Here's how the part is built. I have some questions about the finished solid (model axes, mm). Round coordinates to 2 decimals unless told otherwise and drop trailing zeros. Write item = value, one per line. Start each with the question number.
(1) Will these pins go through, and if not, where does the flat tip stop? pin 1 Ø0.7 at (y, z) = (-0.5, 132.5) entering from -X; pin 2 Ø0.6 at (y, z) = (9, 109) entering from -X; pin 3 Ø1.1 at (y, z) = (0, 100.5) entering from +X.
(2) If we mould it in two halves opening along Y, with no side actions, what happens to faces 1 (the flat face through (-0.1, 2.4, 256.86)), 2 (the cylindrical face through (-1.706, -1.308, 126.632)), 3 (the flat face through (-6, -10, 127))? For each: released by +Y, released by -Y, zero draft, split by the parting line, or undercut.
(3) I need wall thicknesses on line 1 along Y through (x, z) = (3.5, 14.5); line 2 along X through (y, z) = (-4.75, 106); line 3 along X through (y, z) = (2.75, 139.5). Which ranges of each line are inside material? Lowest first, please.
```python
from build123d import *

# Parameters (mm, degrees)
BOSS_EXTRU_1_DEPTH = 256.86


with BuildPart() as part:
    # Esquisse1 → Boss.-Extru.1 (new body)
    with BuildSketch(Plane.XY):
        with BuildLine():
            Line((-3.255887446, 4.528679645), (-5.506192286, 6.778984485))
            ThreePointArc((-5.506192286, 6.778984485), (-5.686636441, 7.686138511), (-4.917588391, 8.199999989))
            Line((-4.917588391, 8.199999989), (-2.799999991, 8.199999989))
            ThreePointArc((-2.799999991, 8.199999989), (-2.587867957, 8.287867955), (-2.499999991, 8.499999989))
            Line((-2.499999991, 8.499999989), (-2.499999991, 9.199999989))
            ThreePointArc((-2.499999991, 9.199999989), (-2.734314566, 9.765685414), (-3.299999991, 9.999999989))
            Line((-3.299999991, 9.999999989), (-7.999999991, 9.999999989))
            ThreePointArc((-7.999999991, 9.999999989), (-9.414213554, 9.414213552), (-9.999999991, 7.999999989))
            Line((-9.999999991, 7.999999989), (-9.999999991, 3.299999989))
            ThreePointArc((-9.999999991, 3.299999989), (-9.765685416, 2.734314564), (-9.199999991, 2.499999989))
            Line((-9.199999991, 2.499999989), (-8.499999991, 2.499999989))
            ThreePointArc((-8.499999991, 2.499999989), (-8.287867957, 2.587867955), (-8.199999991, 2.799999989))
            Line((-8.199999991, 2.799999989), (-8.199999991, 4.917588389))
            ThreePointArc((-8.199999991, 4.917588389), (-7.686138517, 5.686636433), (-6.778984497, 5.506192279))
            Line((-6.778984497, 5.506192279), (-4.528679657, 3.255887439))
            ThreePointArc((-4.528679657, 3.255887439), (-3.878361403, 2.282617393), (-3.650000001, 1.134567096))
            Line((-3.650000001, 1.134567096), (-3.650000001, -1.134567114))
            ThreePointArc((-3.650000001, -1.134567114), (-3.878361403, -2.282617409), (-4.528679656, -3.255887454))
            Line((-4.528679656, -3.255887454), (-6.778984496, -5.506192294))
            ThreePointArc((-6.778984496, -5.506192294), (-7.686138522, -5.686636449), (-8.2, -4.9175884))
            Line((-8.2, -4.9175884), (-8.2, -2.8))
            ThreePointArc((-8.2, -2.8), (-8.287867966, -2.587867966), (-8.5, -2.5))
            Line((-8.5, -2.5), (-9.2, -2.5))
            ThreePointArc((-9.2, -2.5), (-9.765685425, -2.734314575), (-10, -3.3))
            Line((-10, -3.3), (-10, -8))
            ThreePointArc((-10, -8), (-9.414213562, -9.414213562), (-8, -10))
            Line((-8, -10), (-3.3, -10))
            ThreePointArc((-3.3, -10), (-2.734314575, -9.765685425), (-2.5, -9.2))
            Line((-2.5, -9.2), (-2.5, -8.5))
            ThreePointArc((-2.5, -8.5), (-2.587867966, -8.287867966), (-2.8, -8.2))
            Line((-2.8, -8.2), (-4.9175884, -8.2))
            ThreePointArc((-4.9175884, -8.2), (-5.686636444, -7.686138526), (-5.50619229, -6.778984506))
            Line((-5.50619229, -6.778984506), (-3.25588745, -4.528679666))
            ThreePointArc((-3.25588745, -4.528679666), (-2.282617404, -3.878361412), (-1.134567106, -3.650000009))
            Line((-1.134567106, -3.650000009), (1.134567104, -3.650000009))
            ThreePointArc((1.134567104, -3.650000009), (2.282617399, -3.878361412), (3.255887444, -4.528679664))
            Line((3.255887444, -4.528679664), (5.506192284, -6.778984504))
            ThreePointArc((5.506192284, -6.778984504), (5.686636439, -7.686138531), (4.917588389, -8.200000009))
            Line((4.917588389, -8.200000009), (2.799999989, -8.200000009))
            ThreePointArc((2.799999989, -8.200000009), (2.587867955, -8.287867974), (2.499999989, -8.500000009))
            Line((2.499999989, -8.500000009), (2.499999989, -9.200000009))
            ThreePointArc((2.499999989, -9.200000009), (2.734314564, -9.765685434), (3.299999989, -10.000000009))
            Line((3.299999989, -10.000000009), (7.999999989, -10.000000009))
            ThreePointArc((7.999999989, -10.000000009), (9.414213552, -9.414213571), (9.999999989, -8.000000009))
            Line((9.999999989, -8.000000009), (9.999999989, -3.300000009))
            ThreePointArc((9.999999989, -3.300000009), (9.765685414, -2.734314584), (9.199999989, -2.500000009))
            Line((9.199999989, -2.500000009), (8.499999989, -2.500000009))
            ThreePointArc((8.499999989, -2.500000009), (8.287867955, -2.587867974), (8.199999989, -2.800000009))
            Line((8.199999989, -2.800000009), (8.199999989, -4.917588409))
            ThreePointArc((8.199999989, -4.917588409), (7.686138515, -5.686636452), (6.778984495, -5.506192299))
            Line((6.778984495, -5.506192299), (4.528679655, -3.255887459))
            ThreePointArc((4.528679655, -3.255887459), (3.878361401, -2.282617412), (3.649999999, -1.134567115))
            Line((3.649999999, -1.134567115), (3.649999999, 1.134567095))
            ThreePointArc((3.649999999, 1.134567095), (3.878361401, 2.28261739), (4.528679654, 3.255887435))
            Line((4.528679654, 3.255887435), (6.778984494, 5.506192275))
            ThreePointArc((6.778984494, 5.506192275), (7.68613852, 5.68663643), (8.199999998, 4.917588381))
            Line((8.199999998, 4.917588381), (8.199999998, 2.799999981))
            ThreePointArc((8.199999998, 2.799999981), (8.287867964, 2.587867946), (8.499999998, 2.499999981))
            Line((8.499999998, 2.499999981), (9.199999998, 2.499999981))
            ThreePointArc((9.199999998, 2.499999981), (9.765685423, 2.734314556), (9.999999998, 3.299999981))
            Line((9.999999998, 3.299999981), (9.999999998, 7.999999981))
            ThreePointArc((9.999999998, 7.999999981), (9.41421356, 9.414213543), (7.999999998, 9.999999981))
            Line((7.999999998, 9.999999981), (3.299999998, 9.999999981))
            ThreePointArc((3.299999998, 9.999999981), (2.734314573, 9.765685406), (2.499999998, 9.199999981))
            Line((2.499999998, 9.199999981), (2.499999998, 8.499999981))
            ThreePointArc((2.499999998, 8.499999981), (2.587867964, 8.287867946), (2.799999998, 8.199999981))
            Line((2.799999998, 8.199999981), (4.917588398, 8.199999981))
            ThreePointArc((4.917588398, 8.199999981), (5.686636442, 7.686138507), (5.506192288, 6.778984487))
            Line((5.506192288, 6.778984487), (3.255887448, 4.528679647))
            ThreePointArc((3.255887448, 4.528679647), (2.282617402, 3.878361393), (1.134567104, 3.64999999))
            Line((1.134567104, 3.64999999), (-1.134567106, 3.64999999))
            ThreePointArc((-1.134567106, 3.64999999), (-2.282617401, 3.878361392), (-3.255887446, 4.528679645))
        make_face()
        with BuildLine():
            ThreePointArc((-2.15, 0), (0, -2.15), (2.15, 0))
            ThreePointArc((2.15, 0), (0, 2.15), (-2.15, 0))
        make_face(mode=Mode.SUBTRACT)
    extrude(amount=BOSS_EXTRU_1_DEPTH)


solid = part.part
```
Returned:
q1.pin_1 = -3.65
q1.pin_2 = -9.87
q1.pin_3 = 3.65
q2.face_1 = zero draft
q2.face_2 = undercut
q2.face_3 = released by -Y
q3.line_1 = -10 to -8.2, -4.77 to 4.77, 8.2 to 10
q3.line_2 = -10 to -8.2, -6.02 to -3.48, 3.48 to 6.02, 8.2 to 10
q3.line_3 = -9.78 to -8.2, -4.12 to 4.12, 8.2 to 9.78
